from build123d import *

# Parameters (mm, degrees)
BOSS_EXTRUDE1_DEPTH      = 19.05
SKETCH2_R                = 1
SKETCH2_W                = 21.8000072
SKETCH2_H                = 32.97884159
CUT_EXTRUDE1_DEPTH       = 25.515096105
SKETCH3_W                = 33.10001
SKETCH3_H                = 18
CUT_EXTRUDE2_DEPTH       = 3
SKETCH4_W                = 3.3239964
SKETCH4_H                = 19.05
BOSS_EXTRUDE2_DEPTH      = 2
BOSS_EXTRUDE2_DEPTH_BACK = 12.7


with BuildPart() as part:
    # Sketch1 → Boss-Extrude1 (new body, symmetric)
    with BuildSketch(Plane(origin=(0, 0, 0), x_dir=(0, 0, -1), z_dir=(1, 0, 0))):
        Polygon((35, 1.055980791), (35, 7.405980791), (0, 7.405980791), (0, -7.405980791), (35.076175279, -6.515045939), (35, -3.516019209), (5, -4.278019209), (5, 1.055980791), align=None)
        Polygon((0, -17.109115314), (35.322475992, -16.211924424), (35.076175279, -6.515045939), (0, -7.405980791), align=None)
    extrude(amount=BOSS_EXTRUDE1_DEPTH, both=True)

    # Sketch2 → Cut-Extrude1 (cut, through all)
    with BuildSketch(Plane(origin=(0, 7.405980791, 0), x_dir=(1, 0, 0), z_dir=(0, 1, 0))):
        with Locations((-12.5, 31.5)):
            Circle(SKETCH2_R)
        with Locations((12.5, 31.5)):
            Circle(SKETCH2_R)
        with Locations((0, 21.489420795)):
            Rectangle(SKETCH2_W, SKETCH2_H)
    extrude(amount=-CUT_EXTRUDE1_DEPTH, mode=Mode.SUBTRACT)

    # Sketch3 → Cut-Extrude2 (cut)
    with BuildSketch(Plane(origin=(0, 7.405980791, 0), x_dir=(1, 0, 0), z_dir=(0, 1, 0))):
        with Locations((0, 9)):
            Rectangle(SKETCH3_W, SKETCH3_H)
    extrude(amount=-CUT_EXTRUDE2_DEPTH, mode=Mode.SUBTRACT)

    # Sketch4 → Boss-Extrude2 (add, two sides)
    with BuildSketch(Plane(origin=(0, -4.402179099, -0.111815349), x_dir=(1, 0, 0), z_dir=(0, 0.999677576, 0.02539181))) as boss_extrude2_sk:
        with Locations((12.5620018, 25.374437067)):
            Rectangle(SKETCH4_W, SKETCH4_H)
        with Locations((-12.5620018, 25.374437067)):
            Rectangle(SKETCH4_W, SKETCH4_H)
    extrude(amount=BOSS_EXTRUDE2_DEPTH)
    extrude(boss_extrude2_sk.sketch, amount=-BOSS_EXTRUDE2_DEPTH_BACK)


solid = part.part
Input: part model. Units: mm. Frame: model coordinates. A direction names the side the tool comes from. Round coordinates to 2 decimals unless told otherwise and drop trailing zeros. Order: outer loops, then holes, each group sorted by start corner. A loop starts at its lowest first (then second) coordinate and runs counter-clockwise, first axis right, second up. Notation, with made-up numbers: (3, 65.5) - (48, 65.5) arc R27 ccw to (48, 89.5) - close; hole circle Ø8 at (82.25, 34). An arc over 180 degrees is marked (long way). Use a Markdown table: item, result.
1. Section C-C on z = -31.5. Return the cut outline in (x, y), then the cut area to 3 significant figures.
Evaluation:
| item | result |
|---|---|
| outline | (-19.05, -16.31) - (-10.9, -16.31) - (-10.9, -1.6) - (-14.22, -1.6) - (-14.22, -3.6) - (-19.05, -3.6) - close; (-19.05, 1.06) - (-13.5, 1.06) - (-13.5, 7.41) - (-19.05, 7.41) - close; (-11.5, 1.06) - (-10.9, 1.06) - (-10.9, 7.41) - (-11.5, 7.41) - close; (10.9, -16.31) - (19.05, -16.31) - (19.05, -3.6) - (14.22, -3.6) - (14.22, -1.6) - (10.9, -1.6) - close; (10.9, 1.06) - (11.5, 1.06) - (11.5, 7.41) - (10.9, 7.41) - close; (13.5, 1.06) - (19.05, 1.06) - (19.05, 7.41) - (13.5, 7.41) - close |
| area | 298 mm^2 |
2. Section A-A on x = 12.5. Return the cut outline in (y, z), then the cut area to 3 significant figures.
Evaluation:
| item | result |
|---|---|
| outline | (-17.11, 0) - (-16.21, -35.32) - (-1.52, -34.95) - (-2, -15.91) - (-4, -15.96) - (-4.28, -5) - (1.06, -5) - (1.06, -30.5) - (7.41, -30.5) - (7.41, -18) - (4.41, -18) - (4.41, 0) - close; (1.06, -35) - (7.41, -35) - (7.41, -32.5) - (1.06, -32.5) - close |
| area | 667 mm^2 |
3. Material intervals for probe 1 along X at (y, z) = (4.5, -31.5); probe 2 along X at (y, z) = (-14.5, -21.5); probe 3 along Z at (x, y) = (12.5, 6.25), sorted ascending.
Evaluation:
| item | result |
|---|---|
| probe 1 | -19.05 to -13.5, -11.5 to -10.9, 10.9 to 11.5, 13.5 to 19.05 |
| probe 2 | -19.05 to -10.9, 10.9 to 19.05 |
| probe 3 | -35 to -32.5, -30.5 to -18 |
4. Mould query, pull axis Z, two halves, no side actions, for faces 1 (the face through (-16.55, 6, -9)), 2 (the face through (-14, 6, -18)), 3 (the face through (12.37, 4.28, -32.49)). Classes: +Z half, -Z half, draft (parallel to the pull), parting line (faces both ways), or undercut.
Evaluation:
| item | result |
|---|---|
| face 1 | draft |
| face 2 | +Z half |
| face 3 | undercut |
5. First-contact query: pin 1 (4 mm diameter, centred on x = -2, y = 2.5, fed in from -Z); pin 2 (9 mm diameter, centred on x = -16, z = -21, fed in from -Y); pin 3 (12 mm diameter, centred on x = -14, y = -4.5, fed in from -Z). Flat tips, straight axial feed; report the tip coordinate or a pass-through.
Evaluation:
| item | result |
|---|---|
| pin 1 | z = -5 |
| pin 2 | y = -16.69 |
| pin 3 | z = -35.18 |
6. Access query for faces 4 (the face through (15, 1.056, -20)), 5 (the face through (15, 4, -35)), 6 (the face through (10.9, 4, -23)), 7 (the face through (-14.224, -3, -25)). Directions: +Z, -Z, +X, -X, +Y, -Y. A direction counts if a zero-diameter tool reaches every point of the face in a straight line with its end or side. Return the directions, or none.
Evaluation:
| item | result |
|---|---|
| face 4 | -Z, +X, -X |
| face 5 | -Z, +X, -X, +Y |
| face 6 | -Z, +Y, -Y |
| face 7 | -X |
7. Section D-D on y = -9.5. Return the cut outline in (x, z).
Evaluation:
| item | result |
|---|---|
| outline | (-19.05, -35.15) - (-10.9, -35.15) - (-10.9, -5) - (10.9, -5) - (10.9, -35.15) - (19.05, -35.15) - (19.05, 0) - (-19.05, 0) - close |
8. Section B-B on z = -27.5. Return the cut outline in (x, y), then the cut area to 3 significant figures.
Evaluation:
| item | result |
|---|---|
| outline | (-19.05, -16.41) - (-10.9, -16.41) - (-10.9, -1.71) - (-14.22, -1.71) - (-14.22, -3.71) - (-19.05, -3.71) - close; (-19.05, 1.06) - (-10.9, 1.06) - (-10.9, 7.41) - (-19.05, 7.41) - close; (10.9, -16.41) - (19.05, -16.41) - (19.05, -3.71) - (14.22, -3.71) - (14.22, -1.71) - (10.9, -1.71) - close; (10.9, 1.06) - (19.05, 1.06) - (19.05, 7.41) - (10.9, 7.41) - close |
| area | 324 mm^2 |
